Read the model definition and answer for the solid it produces. Units are mm, in the model's axes. A direction names the side the tool comes from. Coordinates: 2 decimals unless noted, no trailing zeros. Loops run counter-clockwise (first coordinate to the right, second up) from the corner with the lowest first, then second, coordinate; pieces in that order, holes last. Notation, with made-up numbers: M -18.5,-38.75 L -13.5,-38.75 A35 cw -13.5,-4.75 Z; hole C 22.25,43 d10. An arc over 180 degrees is marked long. One line per item, written item: value. Start each with the question number.
1. Consider probe 1 along X at (y, z) = (-15, -6.75); probe 2 along Z at (x, y) = (-10, -19); probe 3 along Y at (x, z) = (-13.75, 9.5). Determine where each line is inside the solid, lowest interval first.
2. The part is cut by section B-B (y = -15.5). Write down the section's boundary in (x, z).
3. Flat-ended cylindrical pins translate along their axes: pin 1 (0.8 mm diameter, centred on x = -14.5, z = 3.5, fed in from +Y); pin 2 (4 mm diameter, centred on x = -9, z = -9, fed in from -Y); pin 3 (2 mm diameter, centred on x = -5, z = 1, fed in from -Y). Find the tip coordinate at first contact, or state that the pin passes through.
4. For faces 4 (the face through (-6, 0, 0)), 5 (the face through (-12.42, -5.66, -0.14)), determine the directions among +Z, -Z, +X, -X, +Y, -Y from which every point of the face is accessible in a straight line to the end or side of a thin tool.
5. Determine the mould class of faces 1 (the face through (-14.62, -31.1, 12.14)), 2 (the face through (-9, -13, -10)), 3 (the face through (-9, -13, -13)) for opening direction Z: +Z half, -Z half, draft (parallel to the pull), parting line (faces both ways), or undercut.
6. The part is cut by section A-A (z = 5.5). Write down the section's boundary in (x, y), then the cut area to 3 significant figures.
Autodesk Inventor part; units mm, degrees
ref_plane "YZ Plane" through (0, 0, 0) normal (1, 0, 0) x (0, 1, 0)
ref_plane "XZ Plane" through (0, 0, 0) normal (0, 1, 0) x (-1, 0, 0)
ref_plane "XY Plane" through (0, 0, 0) normal (0, 0, 1) x (1, 0, 0)
sketch "Sketch1" plane through (0, 0, 0) normal (0, 0, 1) x (1, 0, 0)
  line L0 (0, 0) -> (-18, 0)
  line L1 (-18, 0) -> (-18, -32)
  line L2 (-18, -32) -> (0, -32)
  line L3 (0, -32) -> (0, 0)
  dimension "d0" = 18
  dimension "d1" = 32
extrude "Extrusion1" add sketch "Sketch1" along normal mid plane 26
chamfer "Chamfer1" distance 7 angle 45 1 edges at (-18, 0, 0)
chamfer "Chamfer2" distance 13 angle 45 1 edges at (0, -32, 0)
fillet "Fillet1" radius 3 18 edges at (-18, -7, 0) (-11, 0, 0) (0, 0, 0) (0, -9.5, -13) (-5.5, 0, -13) (-14.5, -3.5, -13) (-18, -19.5, -13) (-15.5, -32, -13) (-18, -32, 0) (-15.5, -32, 13) (-18, -19.5, 13) (-14.5, -3.5, 13) (-5.5, 0, 13) (0, -9.5, 13) (0, -19, 0) (-6.5, -25.5, -13) (-13, -32, 0) (-6.5, -25.5, 13)
sketch "Sketch2" plane through (0, 0, 0) normal (0, 0, 1) x (1, 0, 0)
  line L0 (-15, -29) -> (-15, -8.2426)
  line L1 (-14.2426, -29) -> (-15, -29)
  line L2 (-3, -17.7574) -> (-14.2426, -29)
  line L3 (-3, -3) -> (-3, -17.7574)
  line L4 (-9.7574, -3) -> (-3, -3)
  line L5 (-15, -8.2426) -> (-9.7574, -3)
  point P0 (0, 0)
extrude "Extrusion2" cut sketch "Sketch2" along normal mid plane 20
properties part number "Ar620" material "ABS Plastic"
Answer block:
1. probe 1: x = -18 to -15, -3 to 0
1. probe 2: z = -13 to -10, 10 to 13
1. probe 3: y = -31.96 to -28.51, -6.99 to -2.75
2. outline: M -18,-10 A3 ccw -15,-13 L -3,-13 A3 ccw 0,-10 L 0,10 A3 ccw -3,13 L -15,13 A3 ccw -18,10 Z; hole M -15,-10 L -3,-10 L -3,10 L -15,10 Z
3. pin 1: stops at y = -3.1
3. pin 2: stops at y = -30
3. pin 3: stops at y = -25
4. face 4: +Z, -Z, +X, -X, +Y
4. face 5: none
5. face 1: +Z half
5. face 2: undercut
5. face 3: -Z half
6. outline: M -18,-29 A3 ccw -15,-32 L -14.24,-32 A3 ccw -12.12,-31.12 L -0.88,-19.88 A3 ccw 0,-17.76 L 0,-3 A3 ccw -3,0 L -9.76,0 A3 ccw -11.88,-0.88 L -17.12,-6.12 A3 ccw -18,-8.24 Z; hole M -15,-29 L -14.24,-29 L -3,-17.76 L -3,-3 L -9.76,-3 L -15,-8.24 Z
6. area: 227 mm2
